```python
from build123d import *

# Parameters (mm, degrees)
SKETCH1_W                                  = 118
SKETCH1_H                                  = 118
BOSS_EXTRUDE1_DEPTH                        = 4
SKETCH2_W                                  = 118
SKETCH2_H                                  = 118
SKETCH2_W_2                                = 112
SKETCH2_H_2                                = 112
BOSS_EXTRUDE2_DEPTH                        = 30
SKETCH3_W                                  = 16
SKETCH3_H                                  = 16
SKETCH3_R                                  = 2.25
BOSS_EXTRUDE3_DEPTH                        = 6
MIRROR1_AT_THE_SECOND_PLANE_COPY_1_SKETC_W = 16
MIRROR1_AT_THE_SECOND_PLANE_COPY_1_SKETC_H = 16
MIRROR1_AT_THE_SECOND_PLANE_COPY_1_SKETC_R = 2.25
MIRROR1_AT_THE_SECOND_PLANE_COPY_1_DEPTH   = 6
CHAMFER1_SIZE                              = 0.3
FILLET1_R                                  = 8
SKETCH7_W                                  = 3
SKETCH7_H                                  = 24
SKETCH7_W_2                                = 24
SKETCH7_H_2                                = 3
CUT_EXTRUDE1_DEPTH                         = 24
CHAMFER3_SIZE                              = 2.25
BOSS_EXTRUDE4_DEPTH                        = 34
SKETCH9_R                                  = 2.25
CUT_EXTRUDE2_DEPTH                         = 6
MIRROR2_AT_THE_SECOND_PLANE_COPY_1_DEPTH   = 34
MIRROR2_AT_THE_SECOND_PLANE_COPY_2_SKETC_R = 2.25
MIRROR2_AT_THE_SECOND_PLANE_COPY_2_DEPTH   = 6
CHAMFER2_SIZE                              = 0.3
FILLET2_R                                  = 3
FILLET3_R                                  = 3


with BuildPart() as part:
    # Sketch1 → Boss-Extrude1 (new body)
    with BuildSketch(Plane.XY):
        Rectangle(SKETCH1_W, SKETCH1_H)
    extrude(amount=-BOSS_EXTRUDE1_DEPTH)

    # Sketch2 → Boss-Extrude2 (add)
    with BuildSketch(Plane.XY):
        Rectangle(SKETCH2_W, SKETCH2_H)
        Rectangle(SKETCH2_W_2, SKETCH2_H_2, mode=Mode.SUBTRACT)
    extrude(amount=BOSS_EXTRUDE2_DEPTH)

    # Sketch3 → Boss-Extrude3 (add)
    with BuildSketch(Plane.XY):
        with Locations((48, 48)):
            Rectangle(SKETCH3_W, SKETCH3_H)
        with Locations((48, 48)):
            Circle(SKETCH3_R, mode=Mode.SUBTRACT)
    boss_extrude3 = extrude(amount=BOSS_EXTRUDE3_DEPTH)

    # Mirror1: Boss-Extrude3 across plane
    add(boss_extrude3.mirror(Plane(origin=(0, 0, 0), x_dir=(0, 0, 1), z_dir=(1, 0, 0))))

    # Mirror1 at the second plane: Boss-Extrude3 across plane
    add(boss_extrude3.mirror(Plane.ZX))

    # Mirror1 at the second plane copy 1 sketc → Mirror1 at the second plane copy 1 (add)
    with BuildSketch(Plane(origin=(0, 0, 0), x_dir=(-1, 0, 0), z_dir=(0, 0, 1))):
        with Locations((48, 48)):
            Rectangle(MIRROR1_AT_THE_SECOND_PLANE_COPY_1_SKETC_W, MIRROR1_AT_THE_SECOND_PLANE_COPY_1_SKETC_H)
        with Locations((48, 48)):
            Circle(MIRROR1_AT_THE_SECOND_PLANE_COPY_1_SKETC_R, mode=Mode.SUBTRACT)
    extrude(amount=MIRROR1_AT_THE_SECOND_PLANE_COPY_1_DEPTH)

    # Chamfer1
    chamfer1_edges = [part.edges().sort_by_distance(p)[0] for p in [
        (45.75, 48, 6),
        (45.75, -48, 6),
        (-45.75, 48, 6),
        (-45.75, -48, 6),
    ]]
    chamfer(chamfer1_edges, length=CHAMFER1_SIZE)

    # Fillet1
    fillet1_edges = [part.edges().sort_by_distance(p)[0] for p in [
        (40, 40, 3),
        (40, -40, 3),
        (-40, 40, 3),
        (-40, -40, 3),
    ]]
    fillet(fillet1_edges, radius=FILLET1_R)

    # Sketch7 → Cut-Extrude1 (cut)
    with BuildSketch(Plane.XY.offset(30)):
        with Locations((57.5, 27.5)):
            Rectangle(SKETCH7_W, SKETCH7_H)
        with Locations((-27.5, 57.5)):
            Rectangle(SKETCH7_W_2, SKETCH7_H_2)
        with Locations((-57.5, -27.5)):
            Rectangle(SKETCH7_W, SKETCH7_H)
        with Locations((27.5, -57.5)):
            Rectangle(SKETCH7_W_2, SKETCH7_H_2)
    extrude(amount=-CUT_EXTRUDE1_DEPTH, mode=Mode.SUBTRACT)

    # Chamfer3
    chamfer3_edges = [part.edges().sort_by_distance(p)[0] for p in [
        (59, 27.5, 6),
        (59, 39.5, 18),
        (59, 15.5, 18),
        (-27.5, 59, 6),
        (-39.5, 59, 18),
        (-15.5, 59, 18),
        (-59, -27.5, 6),
        (-59, -39.5, 18),
        (-59, -15.5, 18),
        (15.5, -59, 18),
        (27.5, -59, 6),
        (39.5, -59, 18),
    ]]
    chamfer(chamfer3_edges, length=CHAMFER3_SIZE)

    # Sketch8 → Boss-Extrude4 (add)
    with BuildSketch(Plane.XY.offset(30)):
        with BuildLine():
            Line((53, 59), (59, 59))
            Line((59, 59), (59, 53))
            ThreePointArc((59, 53), (63.242640687, 63.242640687), (53, 59))
        make_face()
    boss_extrude4 = extrude(amount=-BOSS_EXTRUDE4_DEPTH)

    # Sketch9 → Cut-Extrude2 (cut)
    with BuildSketch(Plane.XY.offset(30)):
        with Locations((59, 59)):
            Circle(SKETCH9_R)
    cut_extrude2 = extrude(amount=-CUT_EXTRUDE2_DEPTH, mode=Mode.SUBTRACT)

    # Mirror2: Boss-Extrude4, Cut-Extrude2 across plane
    add(boss_extrude4.mirror(Plane(origin=(0, 0, 0), x_dir=(0, 0, 1), z_dir=(1, 0, 0))))
    add(cut_extrude2.mirror(Plane(origin=(0, 0, 0), x_dir=(0, 0, 1), z_dir=(1, 0, 0))), mode=Mode.SUBTRACT)

    # Mirror2 at the second plane: Boss-Extrude4, Cut-Extrude2 across plane
    add(boss_extrude4.mirror(Plane.ZX))
    add(cut_extrude2.mirror(Plane.ZX), mode=Mode.SUBTRACT)

    # Mirror2 at the second plane copy 1 sketc → Mirror2 at the second plane copy 1 (add)
    with BuildSketch(Plane(origin=(0, 0, 30), x_dir=(-1, 0, 0), z_dir=(0, 0, 1))):
        with BuildLine():
            Line((53, 59), (59, 59))
            Line((59, 59), (59, 53))
            ThreePointArc((59, 53), (63.242640687, 63.242640687), (53, 59))
        make_face()
    extrude(amount=-MIRROR2_AT_THE_SECOND_PLANE_COPY_1_DEPTH)

    # Mirror2 at the second plane copy 2 sketc → Mirror2 at the second plane copy 2 (cut)
    with BuildSketch(Plane(origin=(0, 0, 30), x_dir=(-1, 0, 0), z_dir=(0, 0, 1))):
        with Locations((59, 59)):
            Circle(MIRROR2_AT_THE_SECOND_PLANE_COPY_2_SKETC_R)
    extrude(amount=-MIRROR2_AT_THE_SECOND_PLANE_COPY_2_DEPTH, mode=Mode.SUBTRACT)

    # Chamfer2
    chamfer2_edges = [part.edges().sort_by_distance(p)[0] for p in [
        (56.75, 59, 30),
        (56.75, -59, 30),
        (-56.75, 59, 30),
        (-56.75, -59, 30),
    ]]
    chamfer(chamfer2_edges, length=CHAMFER2_SIZE)

    # Fillet2
    fillet2_edges = [part.edges().sort_by_distance(p)[0] for p in [
        (-42.343145751, 42.343145751, 0),
        (-42.343145751, -42.343145751, 0),
        (42.343145751, -42.343145751, 0),
        (42.343145751, 42.343145751, 0),
        (0, 56, 0),
        (40, 52, 0),
        (52, 40, 0),
        (56, 0, 0),
        (52, -40, 0),
        (40, -52, 0),
        (-56, 0, 0),
        (-52, 40, 0),
        (-40, 52, 0),
        (0, -56, 0),
        (-40, -52, 0),
        (-52, -40, 0),
    ]]
    fillet(fillet2_edges, radius=FILLET2_R)

    # Fillet3
    fillet3_edges = [part.edges().sort_by_distance(p)[0] for p in [
        (53, 59, 13),
        (59, 53, 13),
        (59, -53, 13),
        (53, -59, 13),
        (-59, 53, 13),
        (-53, 59, 13),
        (-53, -59, 13),
        (-59, -53, 13),
    ]]
    fillet(fillet3_edges, radius=FILLET3_R)


solid = part.part
```
Input: part model. Units: mm. Frame: model coordinates. A direction names the side the tool comes from. Give positions to 0.01 mm unless a question says otherwise; leave off trailing zeros. Order: outer loops, then holes, each group sorted by start corner. A loop starts at its lowest first (then second) coordinate and runs counter-clockwise, first axis right, second up.
1. Draft query along X for faces 5 (the face through (-56, 12, 16)), 6 (the face through (57, -34, 30)), 7 (the face through (-46.34, -49.52, 2.81)), 8 (the face through (59, -12, 13)). Return one class per face: released by +X, released by -X, zero draft, split by the parting line, or undercut.
Computed:
face 5: undercut
face 6: zero draft
face 7: undercut
face 8: released by +X
2. Line query: probe 1 along X at (y, z) = (1, 26); probe 2 along X at (y, z) = (-48, 2). Output: solid intervals per line, ascending.
Computed:
probe 1: x = -59 to -56, 56 to 59
probe 2: x = -59 to -50.25, -45.75 to -39.83, 39.83 to 45.75, 50.25 to 59
3. Cut plane A-A (z = 26). State how many separate pieces and enclosed holes the cut face has, and give its area (3 significant figures).
Computed:
separate pieces: 4
enclosed holes: 4
area: 1,360 mm2
4. Set-up query: faces 1 (the face through (0.56, 55.1, 0.86)), 2 (the face through (59.566, 52.268, 12.762)), 3 (the face through (63.36, 63.12, 13.24)), 4 (the face through (-59, 11, 13)). Return all of +Z, -Z, +X, -X, +Y, -Y with unobstructed straight access to the full face (end or side cutting, diameter ignored); none if empty.
Computed:
face 1: +Z
face 2: +Z, -Z, +X
face 3: +Z, -Z
face 4: +Z, -Z, -X
5. Cut plane B-B (y = 1). Return loops of the section in (x, z).
Computed:
outline: (-59, -4) - (59, -4) - (59, 30) - (56, 30) - (56, 3) arc R3 cw to (53, 0) - (-53, 0) arc R3 cw to (-56, 3) - (-56, 30) - (-59, 30) - close
6. Pin query (flat end, axial travel): pin 1 Ø6 at (x, y) = (-18.5, 6.5) entering from +Z; pin 2 Ø5 at (y, z) = (24.5, 6) entering from -X; pin 3 Ø1.3 at (x, y) = (-60, -58.5) entering from +Z. Return the tip coordinate at first contact, or that it passes through.
Computed:
pin 1: stops at z = 0
pin 2: stops at x = -59
pin 3: stops at z = 24
7. Cut plane C-C (x = -21). Return loops of the section in (y, z).
Computed:
outline: (-59, -4) - (59, -4) - (59, 3.75) - (56.75, 6) - (56, 6) - (56, 3) arc R3 cw to (53, 0) - (-53, 0) arc R3 cw to (-56, 3) - (-56, 30) - (-59, 30) - close
